Autodesk Inventor part; units mm, degrees
sketch "Sketch1" plane through (0, 0, 0) normal (0, 1, 0) x (-1, 0, 0)
  line L0 (0, 0) -> (-56, 0)
  line L1 (-56, 0) -> (-56, -37)
  line L2 (-56, -37) -> (0, -37)
  line L3 (0, -37) -> (0, 0)
  line L4 (3, -40) -> (-59, -40)
  line L5 (-59, -40) -> (-59, 3)
  line L6 (-59, 3) -> (3, 3)
  line L7 (3, 3) -> (3, -40)
  dimension "d0" = 56
  dimension "d1" = 37
  dimension "d2" = 3
extrude "Extrusion1" add sketch "Sketch1" along normal blind 3 contours L3 L2 L1 L0 | L4 L5 L6 L7
sketch "Sketch2" plane through (0, 3, 0) normal (0, 1, 0) x (1, 0, 0)
  line L0 (-3, -3) -> (59, -3)
  line L1 (59, -3) -> (59, 40)
  line L2 (-3, -3) -> (59, -3)
  line L3 (59, -3) -> (59, 40)
  line L4 (59, 40) -> (-3, 40)
  line L5 (-3, 40) -> (-3, -3)
  line L6 (0, 37) -> (56, 37)
  line L7 (56, 37) -> (56, 0)
  line L8 (56, 0) -> (0, 0)
  line L9 (0, 0) -> (0, 37)
  point P0 (0, 0)
  dimension "d5" = 3
extrude "Extrusion2" add sketch "Sketch2" along normal blind 20
sketch "Sketch3" plane through (0, 3, 0) normal (0, 1, 0) x (1, 0, 0)
  line L0 (1.5, 25) -> (54.5, 25)
  line L1 (54.5, 25) -> (54.5, 0)
  line L2 (54.5, 0) -> (1.5, 0)
  line L3 (1.5, 0) -> (1.5, 25)
  line L4 (0, 37) -> (56, 37)
  line L5 (71.4, 0) -> (-15.4, 0)
  point P0 (0, 0)
  point P1 (28, 37)
  point P2 (28, 25)
  dimension "d8" = 53
  dimension "d9" = 25
  dimension "d10" = 0
  dimension "d12" = 0
extrude "Extrusion3" cut sketch "Sketch3" against normal blind 1.5
sketch "Sketch4" plane through (0, 23, 0) normal (0, 1, 0) x (1, 0, 0)
  line L0 (-3, -3) -> (59, -3)
  line L1 (59, -3) -> (59, 40)
  line L2 (-3, -3) -> (59, -3)
  line L3 (59, -3) -> (59, 40)
  line L4 (59, 40) -> (-3, 40)
  line L5 (-3, 40) -> (-3, -3)
  line L6 (-1.2, 38.2) -> (57.2, 38.2)
  line L7 (57.2, 38.2) -> (57.2, -1.2)
  line L8 (57.2, -1.2) -> (-1.2, -1.2)
  line L9 (-1.2, -1.2) -> (-1.2, 38.2)
  point P0 (0, 0)
  dimension "d15" = 1.8
extrude "Extrusion4" cut sketch "Sketch4" against normal blind 3
fillet "Fillet1" radius 1.5 4 edges at (-3, 10, 3) (59, 10, 3) (59, 10, -40) (-3, 10, -40)
sketch "Sketch5" plane through (59, 0, 1.5) normal (1, 0, 0) x (0, 0, -1)
  point P0 (1.5, 0)
equation "\"d0\" = length_inner"
equation "\"d1\" = width_inner"
equation "\"d2\" = thickness"
equation "\"d3\" = thickness"
equation "\"d5\" = thickness"
equation "\"d6\" = height_inner"
equation "\"d8\" = length_batt"
equation "\"d9\" = width_batt"
equation "\"d13\" = 0.5 * thickness"
equation "\"d15\" = 0.6 * thickness"
equation "\"d16\" = thickness"
equation "\"d18\" = 0.5 * thickness"
equation "\"length_inner\" = 56"
equation "\"width_inner\" = 37"
equation "\"height_inner\" = 20"
equation "\"thickness\" = 3"
equation "\"length_batt\" = 53"
equation "\"width_batt\" = 25"
properties part number "ieee_box"
Input: part model. Units: mm. Frame: model coordinates. A direction names the side the tool comes from. Give positions to 0.01 mm unless a question says otherwise; leave off trailing zeros. Write each loop counter-clockwise with the first axis right and the second up, starting at its lowest first coordinate (ties: lowest second). Pieces come first, ordered by that corner, then holes.
Q1. Section B-B, the plane z = -1. Output: boundary loops of the cut face in (x, y), plus the area to 3 significant figures.
Q2. Section C-C, the plane x = 47. Output: boundary loops of the cut face in (y, z).
Q3. Set-up query: faces 5 (the face through (57.2, 22, -19)), 6 (the face through (59, 10, -18)), 7 (the face through (54.5, 2, -13)), 8 (the face through (28, 22, -38.2)). Return all of +Z, -Z, +X, -X, +Y, -Y with unobstructed straight access to the full face (end or side cutting, diameter ignored); none if empty.
Q4. First-contact query: P1, Ø8, axis at x = 44.5, z = -22.5, coming from the -Y side; P2, Ø1.5, axis at x = 19.5, y = 22, coming from the +Z side; P3, Ø12, axis at x = 7, z = -25, coming from the +Y side; P4, Ø12.5, axis at x = 36.5, z = -17.5, coming from the +Y side. Flat tips, straight axial feed; report the tip coordinate or a pass-through.
Q5. Pull-direction query (X, two-part tool) for faces 1 (the face through (0, 13, -18)), 2 (the face through (28, 10, -40)), 3 (the face through (28, 1.5, -13)), 4 (the face through (58.55, 10.14, 2.57)); classes: pulls with the +X half, pulls with the -X half, needs draft (parallel to the pull), parting line crosses it, or undercut.
Q6. Section D-D, the plane y = 21.5. Output: boundary loops of the cut face in (x, z), plus the area to 3 significant figures.
Q7. Material intervals for probe 1 along X at (y, z) = (16, -21.5); probe 2 along Z at (x, y) = (38, 11.75); probe 3 along X at (y, z) = (21.5, -33), sorted ascending.
Q8. Section A-A, the plane y = 8.75. Output: boundary loops of the cut face in (x, z), plus the area to 3 significant figures.
Filled in:
1. outline: (-3, 0) - (59, 0) - (59, 20) - (57.2, 20) - (57.2, 23) - (56, 23) - (56, 3) - (54.5, 3) - (54.5, 1.5) - (1.5, 1.5) - (1.5, 3) - (0, 3) - (0, 23) - (-1.2, 23) - (-1.2, 20) - (-3, 20) - close
1. area: 216 mm2
2. outline: (0, -40) - (20, -40) - (20, -38.2) - (23, -38.2) - (23, -37) - (3, -37) - (3, -25) - (1.5, -25) - (1.5, 0) - (23, 0) - (23, 1.2) - (20, 1.2) - (20, 3) - (0, 3) - close
3. face 5: +Z, -Z, +X, +Y
3. face 6: +Z, -Z, +X, +Y, -Y
3. face 7: +Y
3. face 8: -Z, +X, -X, +Y
4. P1: stops at y = 0
4. P2: stops at z = 1.2
4. P3: stops at y = 3
4. P4: stops at y = 1.5
5. face 1: undercut
5. face 2: needs draft
5. face 3: undercut
5. face 4: pulls with the +X half
6. outline: (-1.2, -38.2) - (57.2, -38.2) - (57.2, 1.2) - (-1.2, 1.2) - close; hole (0, -37) - (56, -37) - (56, 0) - (0, 0) - close
6. area: 229 mm2
7. probe 1: x = -3 to 0, 56 to 59
7. probe 2: z = -40 to -37, 0 to 3
7. probe 3: x = -1.2 to 0, 56 to 57.2
8. outline: (-3, -38.5) arc R1.5 ccw to (-1.5, -40) - (57.5, -40) arc R1.5 ccw to (59, -38.5) - (59, 1.5) arc R1.5 ccw to (57.5, 3) - (-1.5, 3) arc R1.5 ccw to (-3, 1.5) - close; hole (0, -37) - (56, -37) - (56, 0) - (0, 0) - close
8. area: 592 mm2
